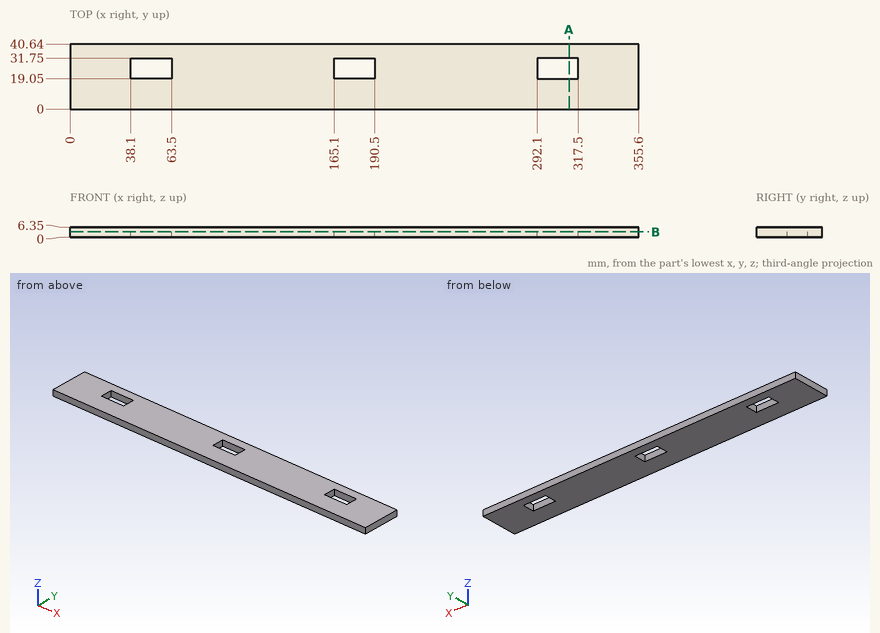
Source: three-view drawing plus pictorial views. Frame: mm from the lowest corner of the part. Round coordinates to 2 decimals unless told otherwise and drop trailing zeros. Loops run counter-clockwise (first coordinate to the right, second up) from the corner with the lowest first, then second, coordinate; pieces in that order, holes last.
Q1. Section B-B, the plane z = 3.25. Return loops of the section in (x, y).
Q2. Section A-A, the plane x = 312. Return loops of the section in (y, z).
Q3. First-contact query: P1, Ø6, axis at x = 170.5, y = 25, coming from the -Z side. Flat tip, straight axial feed; report the tip coordinate or a pass-through.
Q4. Ray query, line 1 (X direction, y = 21, z = 0.5); line 2 (Y direction, x = 48.5, z = 5.5). Return the intervals inside material, ascending.
Solutions:
1. outline: (0, 0) - (355.6, 0) - (355.6, 40.64) - (0, 40.64) - close; hole (38.1, 19.05) - (63.5, 19.05) - (63.5, 31.75) - (38.1, 31.75) - close; hole (165.1, 19.05) - (190.5, 19.05) - (190.5, 31.75) - (165.1, 31.75) - close; hole (292.1, 19.05) - (317.5, 19.05) - (317.5, 31.75) - (292.1, 31.75) - close
2. outline: (0, 0) - (19.05, 0) - (19.05, 6.35) - (0, 6.35) - close; (31.75, 0) - (40.64, 0) - (40.64, 6.35) - (31.75, 6.35) - close
3. P1: passes through
4. line 1: x = 0 to 38.1, 63.5 to 165.1, 190.5 to 292.1, 317.5 to 355.6
4. line 2: y = 0 to 19.05, 31.75 to 40.64
